Geometry check sheet. Reference: the model listing, model coordinates, mm. A direction names the side the tool comes from. Give positions to 0.01 mm unless a question says otherwise; leave off trailing zeros. Write each loop counter-clockwise with the first axis right and the second up, starting at its lowest first coordinate (ties: lowest second). Pieces come first, ordered by that corner, then holes. Notation, with made-up numbers: (75.25, 47) -> (119.25, 47) arc R10 ccw to (119.25, 57) -> close; hole circle Ø6 at (-16, 9.5). An arc over 180 degrees is marked (long way). Write item = value, one per line. Start each with the question number.
1. Cross-section at C-C, the plane x = -3.5. Record the cut outline in (y, z).
2. Set-up check for faces 1 (the flat face through (24, -22, 0)), 2 (the flat face through (-6.831, 31.657, -0.336)), 3 (the flat face through (-24, -22, 0)): record each of +Z, -Z, +X, -X, +Y, -Y from which the full face is reachable in a straight line by a thin tool's end or side.
3. Cross-section at B-B, the plane z = -6. Record the cut outline in (x, y), plus the area to 3 significant figures.
4. Mould release check, pull along X, two halves, no side actions. Record for faces 4 (the flat face through (30.831, -9.912, 0.336)), 5 (the flat face through (3, -1, 24)), 6 (the flat face through (6.831, 31.657, -0.336)): pulls with the +X half, pulls with the -X half, needs draft (parallel to the pull), parting line crosses it, or undercut.
5. Cross-section at A-A, the plane y = 32. Record the cut outline in (x, z).
6. Thickness scan on line 1 along X through (y, z) = (-22, -10); line 2 along X through (y, z) = (31, 2.5); line 3 along Y through (x, z) = (0, 19.5). Record the ranges inside material, lowest first.
7. Depth check by flat-ended pin: P1, Ø17.5, axis at y = -22, z = 11, coming from the +X side; P2, Ø10, axis at y = 19, z = 15, coming from the +X side; P3, Ø5, axis at y = -24.5, z = -6, coming from the -X side. Enter the tip coordinate at first touch or a pass-through.
8. Cross-section at D-D, the plane y = -25. Record the cut outline in (x, z), plus the area to 3 significant figures.
```python
from build123d import *

# Parameters (mm, degrees)
F1_DEPTH = 24
F2_DEPTH = 16
F3_DEPTH = 16
F4_DEPTH = 16


with BuildPart() as f1:
    # F0 (on Top) → F1 (new body, symmetric)
    with BuildSketch(Plane.XY):
        Polygon((24, -13.8564064606), (0, 27.7128129211), (-24, -13.8564064606), align=None)
    extrude(amount=F1_DEPTH, both=True)

    # F2 (add): a face of the model
    f2_faces = [f1.faces().sort_by_distance(p)[0] for p in [
        (0, -13.8564064606, 0),
    ]]
    extrude(f2_faces, amount=F2_DEPTH)

    # F3 (add): a face of the model
    f3_faces = [f1.faces().sort_by_distance(p)[0] for p in [
        (12, 6.9282032303, 0),
    ]]
    extrude(f3_faces, amount=F3_DEPTH)

    # F4 (add): a face of the model
    f4_faces = [f1.faces().sort_by_distance(p)[0] for p in [
        (-12, 6.9282032303, 0),
    ]]
    extrude(f4_faces, amount=F4_DEPTH)


solid = f1.part
```
Answers:
q1.outline = (-29.86, -24) -> (29.73, -24) -> (29.73, 24) -> (-29.86, 24) -> close
q2.face_1 = +Z, -Z, +X, -Y
q2.face_2 = +Z, -Z, +Y
q2.face_3 = +Z, -Z, -X, -Y
q3.outline = (-37.86, -5.86) -> (-24, -13.86) -> (-24, -29.86) -> (24, -29.86) -> (24, -13.86) -> (37.86, -5.86) -> (13.86, 35.71) -> (0, 27.71) -> (-13.86, 35.71) -> close
q3.area = 3,300 mm^2
q4.face_4 = pulls with the +X half
q4.face_5 = needs draft
q4.face_6 = undercut
q5.outline = (-16, -24) -> (-7.43, -24) -> (-7.43, 24) -> (-16, 24) -> close; (7.43, -24) -> (16, -24) -> (16, 24) -> (7.43, 24) -> close
q6.line_1 = -24 to 24
q6.line_2 = -16.58 to -5.69, 5.69 to 16.58
q6.line_3 = -29.86 to 27.71
q7.P1 = 25.05
q7.P2 = 26.39
q7.P3 = -24
q8.outline = (-24, -24) -> (24, -24) -> (24, 24) -> (-24, 24) -> close
q8.area = 2,300 mm^2
